```python
from build123d import *

# Parameters (mm, degrees)
F1_DEPTH  = 100
F2_W      = 5
F2_H      = 10
F3_DEPTH  = 5
F4_R      = 0.9
F5_DEPTH  = 25
F7_DEPTH  = 3.5
F8_DEPTH  = 11.001
F9_SIZE   = 0.5
F10_W     = 11
F10_H     = 5
F10_W_2   = 12
F11_DEPTH = 25
F12_W     = 5
F12_H     = 33
F13_DEPTH = 8
F14_W     = 5
F14_H     = 33
F15_DEPTH = 8
F16_SIZE  = 0.4
F17_R     = 0.5


with BuildPart() as f1:
    # F0 (on Front) → F1 (new body)
    with BuildSketch(Plane.XZ):
        Polygon((2.5, -2.5), (4.75, -2.5), (4.75, 2.5), (10, 2.5), (10, 4.5), (12, 8.5), (10, 8.5), (6, 8.5), (-6, 8.5), (-10, 8.5), (-12, 8.5), (-10, 4.5), (-10, 2.5), (-4.75, 2.5), (-4.75, -2.5), (-2.5, -2.5), (-2.5, 2.5), (2.5, 2.5), align=None)
    extrude(amount=F1_DEPTH)

    # F2 (on face) → F3 (join)
    with BuildSketch(Plane(origin=(0, 0, 2.5), x_dir=(1, 0, 0), z_dir=(0, 0, -1))):
        with Locations((0, 95)):
            Rectangle(F2_W, F2_H)
        Polygon((-2.5, 50), (-2.5, 45), (2.5, 45), (2.5, 50), (2.5, 55), (-2.5, 55), align=None)
        with Locations((0, 5)):
            Rectangle(F2_W, F2_H)
    extrude(amount=F3_DEPTH)

    # F4 (on face) → F5 (cut)
    with BuildSketch(Plane.YZ.offset(4.75)):
        with Locations((-85, 0)):
            Circle(F4_R)
        with Locations((-40, 0)):
            Circle(F4_R)
        with BuildLine():
            ThreePointArc((-14.1, 0), (-15, 0.9), (-15.9, 0))
            Line((-15.9, 0), (-14.1, 0))
        make_face()
        with BuildLine():
            Line((-14.1, 0), (-15.9, 0))
            ThreePointArc((-15.9, 0), (-15, -0.9), (-14.1, 0))
        make_face()
        with Locations((-60, 0)):
            Circle(F4_R)
    extrude(amount=-F5_DEPTH, mode=Mode.SUBTRACT)

    # F6 (on face) → F7 (cut)
    with BuildSketch(Plane.XY.offset(8.5)):
        with BuildLine():
            ThreePointArc((0, -92), (-3, -95), (0, -98))
            Line((0, -98), (0, -96.75))
            ThreePointArc((0, -96.75), (-1.75, -95), (0, -93.25))
            Line((0, -93.25), (0, -92))
        make_face()
        with BuildLine():
            ThreePointArc((0, -2), (-3, -5), (0, -8))
            Line((0, -8), (0, -6.75))
            ThreePointArc((0, -6.75), (-1.75, -5), (0, -3.25))
            Line((0, -3.25), (0, -2))
        make_face()
        with BuildLine():
            Line((0, -6.75), (0, -8))
            ThreePointArc((0, -8), (2.1213203436, -7.1213203436), (3, -5))
            ThreePointArc((3, -5), (2.1213203436, -2.8786796564), (0, -2))
            Line((0, -2), (0, -3.25))
            ThreePointArc((0, -3.25), (1.2374368671, -3.7625631329), (1.75, -5))
            ThreePointArc((1.75, -5), (1.2374368671, -6.2374368671), (0, -6.75))
        make_face()
        with BuildLine():
            ThreePointArc((0, -47), (-3, -50), (0, -53))
            Line((0, -53), (0, -51.75))
            ThreePointArc((0, -51.75), (-1.75, -50), (0, -48.25))
            Line((0, -48.25), (0, -47))
        make_face()
        with BuildLine():
            Line((0, -51.75), (0, -53))
            ThreePointArc((0, -53), (2.1213203436, -52.1213203436), (3, -50))
            ThreePointArc((3, -50), (2.1213203436, -47.8786796564), (0, -47))
            Line((0, -47), (0, -48.25))
            ThreePointArc((0, -48.25), (1.2374368671, -48.7625631329), (1.75, -50))
            ThreePointArc((1.75, -50), (1.2374368671, -51.2374368671), (0, -51.75))
        make_face()
        with BuildLine():
            Line((0, -96.75), (0, -98))
            ThreePointArc((0, -98), (2.1213203436, -97.1213203436), (3, -95))
            ThreePointArc((3, -95), (2.1213203436, -92.8786796564), (0, -92))
            Line((0, -92), (0, -93.25))
            ThreePointArc((0, -93.25), (1.2374368671, -93.7625631329), (1.75, -95))
            ThreePointArc((1.75, -95), (1.2374368671, -96.2374368671), (0, -96.75))
        make_face()
    extrude(amount=-F7_DEPTH, mode=Mode.SUBTRACT)

    # F8 (cut, through all): faces of the model
    f8_faces = [f1.faces().sort_by_distance(p)[0] for p in [
        (0, -5, 8.5),
        (0, -50, 8.5),
        (0, -95, 8.5),
    ]]
    extrude(f8_faces, amount=-F8_DEPTH, mode=Mode.SUBTRACT)

    # F9
    f9_edges = [f1.edges().sort_by_distance(p)[0] for p in [
        (0, -2, 8.5),
        (0, -47, 8.5),
        (0, -92, 8.5),
        (0, -6.75, 5),
        (0, -51.75, 5),
        (0, -96.75, 5),
        (0, -96.75, -2.5),
        (0, -51.75, -2.5),
        (0, -6.75, -2.5),
    ]]
    chamfer(f9_edges, length=F9_SIZE)

    # F10 (on face) → F11 (cut)
    with BuildSketch(Plane(origin=(-4.75, 0, 0), x_dir=(0, -1, 0), z_dir=(-1, 0, 0))):
        with Locations((5.5, 0)):
            Rectangle(F10_W, F10_H)
        with Locations((50, 0)):
            Rectangle(F10_W_2, F10_H)
        with Locations((94.5, 0)):
            Rectangle(F10_W, F10_H)
    extrude(amount=-F11_DEPTH, mode=Mode.SUBTRACT)

    # F12 (on face) → F13 (cut)
    with BuildSketch(Plane(origin=(0, 0, -2.5), x_dir=(1, 0, 0), z_dir=(0, 0, -1))):
        with Locations((0, 72.5)):
            Rectangle(F12_W, F12_H)
    extrude(amount=-F13_DEPTH, mode=Mode.SUBTRACT)

    # F14 (on face) → F15 (cut)
    with BuildSketch(Plane(origin=(0, 0, -2.5), x_dir=(1, 0, 0), z_dir=(0, 0, -1))):
        with Locations((0, 27.5)):
            Rectangle(F14_W, F14_H)
    extrude(amount=-F15_DEPTH, mode=Mode.SUBTRACT)

    # F16
    f16_edges = [f1.edges().sort_by_distance(p)[0] for p in [
        (-3.625, -11, -2.5),
        (-2.5, -27.5, -2.5),
        (-3.625, -44, -2.5),
        (-4.75, -27.5, -2.5),
        (4.75, -27.5, -2.5),
        (3.625, -44, -2.5),
        (2.5, -27.5, -2.5),
        (3.625, -11, -2.5),
        (4.75, -72.5, -2.5),
        (3.625, -89, -2.5),
        (2.5, -72.5, -2.5),
        (3.625, -56, -2.5),
        (-3.625, -56, -2.5),
        (-2.5, -72.5, -2.5),
        (-3.625, -89, -2.5),
        (-4.75, -72.5, -2.5),
        (0, -44, 5.5),
        (-2.5, -27.5, 5.5),
        (0, -11, 5.5),
        (2.5, -27.5, 5.5),
        (0, -89, 5.5),
        (-2.5, -72.5, 5.5),
        (0, -56, 5.5),
        (2.5, -72.5, 5.5),
    ]]
    chamfer(f16_edges, length=F16_SIZE)

    # F17
    f17_edges = [f1.edges().sort_by_distance(p)[0] for p in [
        (12, -50, 8.5),
        (-12, -50, 8.5),
    ]]
    fillet(f17_edges, radius=F17_R)


solid = f1.part
```
Work out the finished part from the listing and answer in its coordinate system (mm). A direction names the side the tool comes from. Give positions to 0.01 mm unless a question says otherwise; leave off trailing zeros. Loops run counter-clockwise (first coordinate to the right, second up) from the corner with the lowest first, then second, coordinate; pieces in that order, holes last. Notation, with made-up numbers: M -3,63.25 L 31,63.25 A33 ccw 31,99.25 Z; hole C -0.75,70 d10. An arc over 180 degrees is marked long. One line per item, written item: value. Start each with the question number.
1. Find section C-C (x = 7.75). Give the vertices of the cut face in (y, z), and give its area (3 significant figures).
2. Determine the mould class of faces 1 (the face through (-4.75, -72, 0)), 2 (the face through (-4, -11, 0)), 3 (the face through (4, -44, 0)), 4 (the face through (-3.61, -84.14, 0.27)) for opening direction Y: released by +Y, released by -Y, zero draft, split by the parting line, or undercut.
3. Each of these flat-tipped pins is pushed along its axis until it touches: P1, Ø1.4, axis at y = -15, z = 0, coming from the +X side; P2, Ø2.5, axis at y = -40, z = 0, coming from the -X side; P3, Ø3.5, axis at y = -79, z = 0.5, coming from the +X side; P4, Ø2.5, axis at x = -3.5, z = -0.5, coming from the -Y side. Where does it stop, or does it pass through?
4. Which of the six approach directions +Z, -Z, +X, -X, +Y, -Y give full straight-line access (tool end or side, diameter ignored) to faces 5 (the face through (10, -49, 3)), 6 (the face through (-4.75, -27, 0)), 7 (the face through (0, -89, 4))?
5. Find section A-A (y = -15). State how many separate pieces and enclosed holes the cut face has, and give its area (3 significant figures).
6. Find section B-B (y = -83). Give the vertices of the cut face in (x, z), and give its area (3 significant figures).
7. Find the intervals of material crossed by probe 1 along Z at (x, y) = (-3, -85); probe 2 along X at (y, z) = (-24.5, 0.75); probe 3 along X at (y, z) = (-26.5, 4), in increasing order.
Reported:
1. outline: M -100,2.5 L 0,2.5 L 0,8.5 L -100,8.5 Z
1. area: 600 mm²
2. face 1: zero draft
2. face 2: released by +Y
2. face 3: undercut
2. face 4: undercut
3. P1: passes through
3. P2: stops at x = -4.75
3. P3: stops at x = 4.75
3. P4: stops at y = -89
4. face 5: -Z, +X, +Y, -Y
4. face 6: -Z, -X, +Y, -Y
4. face 7: -Z
5. separate pieces: 3
5. enclosed holes: 0
5. area: 127 mm²
6. outline: M -11.64,7.78 L -10,4.5 L -10,2.5 L -4.75,2.5 L -4.75,-2.1 L -4.35,-2.5 L -2.9,-2.5 L -2.5,-2.1 L -2.5,5.1 L -2.1,5.5 L 2.1,5.5 L 2.5,5.1 L 2.5,-2.1 L 2.9,-2.5 L 4.35,-2.5 L 4.75,-2.1 L 4.75,2.5 L 10,2.5 L 10,4.5 L 11.64,7.78 A0.5 ccw 11.19,8.5 L -11.19,8.5 A0.5 ccw Z
6. area: 135 mm²
7. probe 1: z = -2.5 to -0.9, 0.9 to 8.5
7. probe 2: x = -4.75 to -2.5, 2.5 to 4.75
7. probe 3: x = -10 to -2.5, 2.5 to 10
